Autodesk Inventor part; units mm, degrees
ref_plane "YZ Plane" through (0, 0, 0) normal (1, 0, 0) x (0, 1, 0)
ref_plane "XZ Plane" through (0, 0, 0) normal (0, 1, 0) x (-1, 0, 0)
ref_plane "XY Plane" through (0, 0, 0) normal (0, 0, 1) x (1, 0, 0)
sketch "Skizze1" plane through (0, 0, 0) normal (0, 0, 1) x (1, 0, 0)
  line L0 (-87.5, -55.5) -> (87.5, -55.5)
  line L1 (87.5, -55.5) -> (87.5, 55.5)
  line L2 (87.5, 55.5) -> (-87.5, 55.5)
  line L3 (-87.5, 55.5) -> (-87.5, -55.5)
  line L4 (-87.5, -55.5) -> (87.5, 55.5) construction
  line L5 (87.5, -55.5) -> (-87.5, 55.5) construction
  point P0 (0, 0)
  dimension "d0" = 175
  dimension "d1" = 111
extrude "Extrusion1" add sketch "Skizze1" along normal blind 15
sketch "Skizze2" plane through (0, 0, 15) normal (0, 0, 1) x (1, 0, 0)
  line L0 (87.5, 55.5) -> (-87.5, 55.5)
  line L1 (-87.5, 55.5) -> (-52.5, 55.5) construction
  line L2 (-52.5, 55.5) -> (-52.5, 29) construction
  line L3 (-52.5, 29) -> (-87.5, 29) construction
  line L4 (-87.5, 29) -> (-87.5, 55.5) construction
  line L5 (87.5, 55.5) -> (52.5, 55.5) construction
  line L6 (52.5, 55.5) -> (52.5, 18) construction
  line L7 (52.5, 18) -> (87.5, 18) construction
  line L8 (87.5, 18) -> (87.5, 55.5) construction
  circle A0 centre (-52.5, 29) radius 1
  circle A1 centre (52.5, 18) radius 1
  point P0 (0, 0)
  dimension "d4" = 35
  dimension "d5" = 26.5
  dimension "d6" = 35
  dimension "d7" = 37.5
  dimension "d8" = 2
  dimension "d9" = 2
extrude "Extrusion2" cut sketch "Skizze2" against normal blind 19.5
chamfer "Fasen1" distance 6 angle 45 4 edges at (-87.5, 0, 15) (0, -55.5, 15) (87.5, 0, 15) (0, 55.5, 15)
properties part number "sf_Wood_Base_1"
Model file for the job. Use its own axes, mm. Coordinates: 2 decimals unless noted, no trailing zeros. Loops run counter-clockwise (first coordinate to the right, second up) from the corner with the lowest first, then second, coordinate; pieces in that order, holes last. Notation, with made-up numbers: (87, 50.5) - (106, 50.5) arc R8 cw to (106, 62.5) - close; hole circle Ø4 at (-9.75, 3). An arc over 180 degrees is marked (long way). Write item = value, one per line. Start each with the question number.
Item 1: Drop a flat-ended pin along its axis: pin 1 Ø3 at (x, z) = (33.5, 13) entering from -Y. Give the stop position or say it passes through.
Item 2: Wall check: probe 1 along Y at (x, z) = (-52.5, 3.5); probe 2 along Y at (x, z) = (52.5, 6.25); probe 3 along Y at (x, z) = (-23, 13). Give the ranges that are in metal, low to high. Write a range as [from, to].
Item 3: Saw through at A-A, the plane x = -69. List the corners of the cut face in (y, z).
Answers:
q1.pin_1 = -53
q2.probe_1 = [-55.5, 28], [30, 55.5]
q2.probe_2 = [-55.5, 17], [19, 55.5]
q2.probe_3 = [-51.5, 51.5]
q3.outline = (-55.5, 0) - (55.5, 0) - (55.5, 9) - (49.5, 15) - (-49.5, 15) - (-55.5, 9) - close
